from build123d import *

# Parameters (mm, degrees)
BOSS_EXTRUDE1_DEPTH = 4
FILLET1_R           = 2
FILLET2_R           = 2


with BuildPart() as part:
    # Sketch1 → Boss-Extrude1 (new body)
    with BuildSketch(Plane.XY):
        with BuildLine():
            Line((54, 18), (54, -14))
            ThreePointArc((54, -14), (52.242640687, -18.242640687), (48, -20))
            Line((48, -20), (-44, -20))
            ThreePointArc((-44, -20), (-48.242640687, -18.242640687), (-50, -14))
            Line((-50, -14), (-50, 18))
            ThreePointArc((-50, 18), (-48.242640687, 22.242640687), (-44, 24))
            Line((-44, 24), (48, 24))
            ThreePointArc((48, 24), (52.242640687, 22.242640687), (54, 18))
        make_face()
        with BuildLine():
            Line((50, 18), (50, -14))
            ThreePointArc((50, -14), (49.414213562, -15.414213562), (48, -16))
            Line((48, -16), (-44, -16))
            ThreePointArc((-44, -16), (-45.414213562, -15.414213562), (-46, -14))
            Line((-46, -14), (-46, 18))
            ThreePointArc((-46, 18), (-45.414213562, 19.414213562), (-44, 20))
            Line((-44, 20), (48, 20))
            ThreePointArc((48, 20), (49.414213562, 19.414213562), (50, 18))
        make_face(mode=Mode.SUBTRACT)
    extrude(amount=BOSS_EXTRUDE1_DEPTH)

    # Fillet1
    fillet1_edges = [part.edges().sort_by_distance(p)[0] for p in [
        (-48.242640687, 22.242640687, 4),
        (-50, 2, 4),
        (-48.242640687, -18.242640687, 4),
        (2, -20, 4),
        (52.242640687, -18.242640687, 4),
        (-45.414213562, 19.414213562, 4),
        (-46, 2, 4),
        (-45.414213562, -15.414213562, 4),
        (2, -16, 4),
        (49.414213562, -15.414213562, 4),
        (50, 2, 4),
        (49.414213562, 19.414213562, 4),
        (54, 2, 4),
        (2, 20, 4),
        (52.242640687, 22.242640687, 4),
        (2, 24, 4),
    ]]
    fillet(fillet1_edges, radius=FILLET1_R - 0.0001)  # a hair under: the kernel refuses the full size

    # Fillet2
    fillet2_edges = [part.edges().sort_by_distance(p)[0] for p in [
        (49.414213562, 19.414213562, 0),
        (50, 2, 0),
        (49.414213562, -15.414213562, 0),
        (2, -16, 0),
        (-45.414213562, -15.414213562, 0),
        (-46, 2, 0),
        (-45.414213562, 19.414213562, 0),
        (2, 20, 0),
        (2, 24, 0),
        (-48.242640687, 22.242640687, 0),
        (-50, 2, 0),
        (-48.242640687, -18.242640687, 0),
        (2, -20, 0),
        (52.242640687, -18.242640687, 0),
        (54, 2, 0),
        (52.242640687, 22.242640687, 0),
    ]]
    fillet(fillet2_edges, radius=FILLET2_R - 0.0001)  # a hair under: the kernel refuses the full size


solid = part.part
Can you work these out from the model? Positions are in its coordinate system, mm. A direction names the side the tool comes from. Coordinates: 2 decimals unless noted, no trailing zeros. Loops run counter-clockwise (first coordinate to the right, second up) from the corner with the lowest first, then second, coordinate; pieces in that order, holes last. Notation, with made-up numbers: (-38, -8.5) - (-7, -8.5) arc R30 ccw to (-7, 16.5) - close; hole circle Ø6 at (10.5, 43). An arc over 180 degrees is marked (long way). Put each result on its own line as item: value. Start each with the question number.
Item 1: For pin 1 (1 mm diameter, centred on y = -13.5, z = 1, fed in from -X); pin 2 (2 mm diameter, centred on x = 40, z = 3.5, fed in from -Y), each with a flat end and sliding along its axis, tell me the tip position at first contact or that it passes through.
Item 2: If we mould it in two halves opening along X, with no side actions, what happens to faces 1 (the face through (-49.4, 2.22, 0.57)), 2 (the face through (53.4, 1.78, 0.57)), 3 (the face through (-46.57, 2.22, 3.4))? For each: +X half, -X half, draft (parallel to the pull), parting line (faces both ways), or undercut.
Item 3: Suppose I cut it at C-C (z = 3.3). Please give me the cut outline in (x, y).
Item 4: If I drill on line 1 along Y through (x, z) = (48, 2); line 2 along X through (y, z) = (9, 3.5); line 3 along Y through (x, z) = (42.5, 0.75), over which ranges is the centre line in solid material (lowest first)?
Item 5: Which directions (+Z, -Z, +X, -X, +Y, -Y) give clear straight access to the entire face, cutting with the end or side of a thin tool? Please do faces 4 (the face through (50.6, 1.78, 0.57)), 5 (the face through (50.57, 1.78, 3.4)), 6 (the face through (1.36, -19.4, 0.57)).
Here are the results:
1. pin 1: x = -49.94
1. pin 2: y = -19.94
2. face 1: -X half
2. face 2: +X half
2. face 3: undercut
3. outline: (-49.52, -14) arc R5.52 ccw to (-44, -19.52) - (48, -19.52) arc R5.52 ccw to (53.52, -14) - (53.52, 18) arc R5.52 ccw to (48, 23.52) - (-44, 23.52) arc R5.52 ccw to (-49.52, 18) - close; hole (-46.48, -14) arc R2.48 ccw to (-44, -16.48) - (48, -16.48) arc R2.48 ccw to (50.48, -14) - (50.48, 18) arc R2.48 ccw to (48, 20.48) - (-44, 20.48) arc R2.48 ccw to (-46.48, 18) - close
4. line 1: -20 to -16, 20 to 24
4. line 2: -49.32 to -46.68, 50.68 to 53.32
4. line 3: -19.56 to -16.44, 20.44 to 23.56
5. face 4: -Z
5. face 5: +Z
5. face 6: -Z, +X, -X, -Y
